The figure shows three views and two pictorial views of one solid part (mm, origin at its lowest corner). Answer the questions. Round coordinates to 2 decimals unless told otherwise and drop trailing zeros. Write each loop counter-clockwise with the first axis right and the second up, starting at its lowest first coordinate (ties: lowest second). Pieces come first, ordered by that corner, then holes.
Item 1: This flat-tipped pin is pushed along its axis until it touches: pin 1 (10 mm diameter, centred on x = 224.5, z = 15.5, fed in from -Y). Where does it stop, or does it pass through?
Item 2: Find section C-C on z = 19.25. Give the vertices of the cut face in (x, y).
Item 3: Find the intervals of material crossed by probe 1 along Y at (x, z) = (254, 17.75); probe 2 along Y at (x, z) = (329.5, 9); probe 3 along X at (y, z) = (136, 5.75), in increasing order.
Item 4: Find section A-A on x = 254. Give the vertices of the cut face in (y, z), then the cut area to 3 significant figures.
Item 5: Find section D-D on x = 31.5. Give the vertices of the cut face in (y, z).
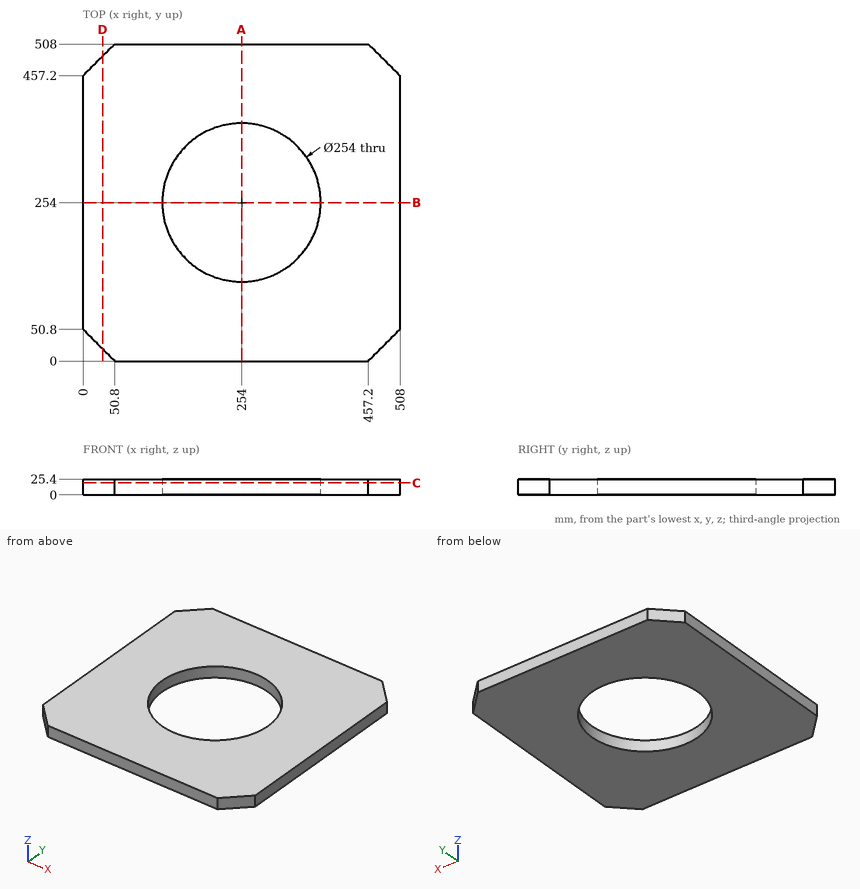
Check values:
1. pin 1: stops at y = 0
2. outline: (0, 50.8) - (50.8, 0) - (457.2, 0) - (508, 50.8) - (508, 457.2) - (457.2, 508) - (50.8, 508) - (0, 457.2) - close; hole circle Ø254 at (254, 254)
3. probe 1: y = 0 to 127, 381 to 508
3. probe 2: y = 0 to 151.88, 356.12 to 508
3. probe 3: x = 0 to 207.04, 300.96 to 508
4. outline: (0, 0) - (127, 0) - (127, 25.4) - (0, 25.4) - close; (381, 0) - (508, 0) - (508, 25.4) - (381, 25.4) - close
4. area: 6,450 mm2
5. outline: (19.3, 0) - (488.7, 0) - (488.7, 25.4) - (19.3, 25.4) - close
